```python
from build123d import *

# Parameters (mm, degrees)
F0_R     = 3
F1_DEPTH = 30
F3_R     = 4
F3_R_2   = 3
F4_DEPTH = 6
F2_R     = 4
F2_R_2   = 3
F5_DEPTH = 8


with BuildPart() as f1:
    # F0 (on Front) → F1 (new body, symmetric)
    with BuildSketch(Plane.XZ):
        Circle(F0_R)
    extrude(amount=F1_DEPTH, both=True)

    # F3 (on face) → F4 (join)
    with BuildSketch(Plane(origin=(0, 30, 0), x_dir=(-1, 0, 0), z_dir=(0, 1, 0))):
        Circle(F3_R)
        Circle(F3_R_2, mode=Mode.SUBTRACT)
        Circle(F3_R_2)
    extrude(amount=F4_DEPTH)

    # F2 (on face) → F5 (join)
    with BuildSketch(Plane.XZ.offset(30)):
        Circle(F2_R)
        Circle(F2_R_2, mode=Mode.SUBTRACT)
        Circle(F2_R_2)
    extrude(amount=F5_DEPTH)


solid = f1.part
```
Read the model definition and answer for the solid it produces. Units are mm, in the model's axes. A direction names the side the tool comes from. Give positions to 0.01 mm unless a question says otherwise; leave off trailing zeros. Write each loop counter-clockwise with the first axis right and the second up, starting at its lowest first coordinate (ties: lowest second). Pieces come first, ordered by that corner, then holes. Notation, with made-up numbers: (-0.75, -27) -> (7.25, -27) arc R12 ccw to (7.25, -6) -> close; hole circle Ø3 at (33.25, 34). An arc over 180 degrees is marked (long way). Answer as a JSON object with one key per item and string values.
1) Flat-ended cylindrical pins translate along their axes: pin 1 Ø3 at (y, z) = (7.5, -0.5) entering from +X; pin 2 Ø2 at (y, z) = (-19.5, -3) entering from +X. Find the tip coordinate at first contact, or state that the pin passes through.
Findings below:
{"pin 1": "stops at x = 3", "pin 2": "stops at x = 2.24"}
2) For a pull along Y with two mould halves and no side action, classify faces 3 (the flat face through (0, -38, 0)), 4 (the flat face through (-1, 30, 3)), 5 (the flat face through (0, 36, 0)) as pulls with the +Y half, pulls with the -Y half, needs draft (parallel to the pull), parting line crosses it, or undercut.
Findings below:
{"face 3": "pulls with the -Y half", "face 4": "undercut", "face 5": "pulls with the +Y half"}
3) Section B-B on x = 0 is taken. Write down the section's boundary in (y, z), then the cut area to 3 significant figures.
Findings below:
{"outline": "(-38, -4) -> (-30, -4) -> (-30, -3) -> (30, -3) -> (30, -4) -> (36, -4) -> (36, 4) -> (30, 4) -> (30, 3) -> (-30, 3) -> (-30, 4) -> (-38, 4) -> close", "area": "472 mm^2"}
4) Section C-C on y = 23 is taken. Write down the section's boundary in (x, z).
Findings below:
{"outline": "circle Ø6 at (0, 0)"}
5) A tool of negligible diameter and unlimited length cuts with its end or side. For faces 1 (the cylindrical face through (0.867, 32.958, -3.905)), 2 (the cylindrical face through (-3, 0, 0)), from which of +Z, -Z, +X, -X, +Y, -Y can it reach the whole face along a straight path? Write none if from no direction.
Findings below:
{"face 1": "+Y, -Y", "face 2": "none"}
6) Straight lines are drawn through the part: probe 1 along Y at (x, z) = (-2.5, 2); probe 2 along X at (y, z) = (-17.5, -0.25); probe 3 along Z at (x, y) = (2.5, -4). For each, find the intervals that lie inside material, in ascending order. Write a range as from..to.
Findings below:
{"probe 1": "y = -38..-30, 30..36", "probe 2": "x = -2.99..2.99", "probe 3": "z = -1.66..1.66"}
7) Section A-A on z = 0 is taken. Write down the section's boundary in (x, y).
Findings below:
{"outline": "(-4, -38) -> (4, -38) -> (4, -30) -> (3, -30) -> (3, 30) -> (4, 30) -> (4, 36) -> (-4, 36) -> (-4, 30) -> (-3, 30) -> (-3, -30) -> (-4, -30) -> close"}
